Source: CAD feature listing. Evaluate the final solid. Frame: model axes, mm. A direction names the side the tool comes from. Give positions to 0.01 mm unless a question says otherwise; leave off trailing zeros. Order: outer loops, then holes, each group sorted by start corner. A loop starts at its lowest first (then second) coordinate and runs counter-clockwise, first axis right, second up.
Autodesk Inventor part; units mm, degrees
ref_plane "YZ Plane" through (0, 0, 0) normal (1, 0, 0) x (0, 1, 0)
ref_plane "XZ Plane" through (0, 0, 0) normal (0, 1, 0) x (-1, 0, 0)
ref_plane "XY Plane" through (0, 0, 0) normal (0, 0, 1) x (1, 0, 0)
sketch "Sketch1" plane through (0, 0, 0) normal (0, 0, 1) x (1, 0, 0)
  line L0 (-60.5, 11) -> (-54, 11)
  line L1 (-54, 11) -> (-54, 9)
  line L2 (-54, 9) -> (54, 9)
  line L3 (54, 9) -> (54, 11)
  line L4 (54, 11) -> (60.5, 11)
  line L5 (60.5, 11) -> (60.5, 22)
  line L6 (60.5, 22) -> (58.5, 22)
  line L7 (58.5, 22) -> (52.5, 16)
  line L8 (52.5, 16) -> (-52.5, 16)
  line L9 (-52.5, 16) -> (-58.5, 22)
  line L10 (-58.5, 22) -> (-60.5, 22)
  line L11 (-60.5, 22) -> (-60.5, 11)
  line L12 (-84.7, 0) -> (84.7, 0)
  point P0 (0, 0)
  point P1 (0, 16)
  point P2 (0, 9)
  dimension "d0" = 11
  dimension "d1" = 6.5
  dimension "d2" = 9
  dimension "d4" = 105
  dimension "d6" = 2
  dimension "d7" = 16
  dimension "d8" = 22
revolve "Revolution1" add sketch "Sketch1" angle 360 about axis through (-10, 0, 0) along (1, 0, 0)
properties part number "Riiserolle"
1) First-contact query: pin 1 Ø2 at (x, y) = (-46, 1) entering from +Z; pin 2 Ø6 at (x, z) = (40, 8) entering from -Y; pin 3 Ø17.5 at (y, z) = (5, 3.5) entering from -X; pin 4 Ø8 at (x, z) = (27.5, -10) entering from -Y. Flat tips, straight axial feed; report the tip coordinate or a pass-through.
Checks:
pin 1: stops at z = 16
pin 2: stops at y = -15.2
pin 3: stops at x = -60.5
pin 4: stops at y = -14.83
2) Section query C-C on x = 40. Output: boundary loops of the cut face in (y, z).
Checks:
outline: circle Ø32 at (0, 0); hole circle Ø18 at (0, 0)
3) Section query A-A on z = 0. Output: boundary loops of the cut face in (x, y), and give its area (3 significant figures).
Checks:
outline: (-60.5, -22) - (-58.5, -22) - (-52.5, -16) - (52.5, -16) - (58.5, -22) - (60.5, -22) - (60.5, -11) - (54, -11) - (54, -9) - (-54, -9) - (-54, -11) - (-60.5, -11) - close; (-60.5, 11) - (-54, 11) - (-54, 9) - (54, 9) - (54, 11) - (60.5, 11) - (60.5, 22) - (58.5, 22) - (52.5, 16) - (-52.5, 16) - (-58.5, 22) - (-60.5, 22) - close
area: 1,760 mm2
4) Pull-direction query (Z, two-part tool) for faces 1 (the face through (-59.514, -4.769, 21.477)), 2 (the face through (0.756, -1.172, 8.923)), 3 (the face through (60.5, 5, 10)); classes: +Z half, -Z half, draft (parallel to the pull), parting line (faces both ways), or undercut.
Checks:
face 1: parting line
face 2: undercut
face 3: draft
5) Reachability of faces 4 (the face through (57.3, -2.38, -10.74)), 5 (the face through (-60.5, 5, 10)), 6 (the face through (-57.2, -2.38, -10.74)), 7 (the face through (-52.875, 15.619, -4.919)) from +Z, -Z, +X, -X, +Y, -Y: full face, straight path, thin tool, end or side. Return the list, or none.
Checks:
face 4: +X
face 5: +Z, -Z, -X, +Y, -Y
face 6: -X
face 7: none
6) Ray query, L1, parallel to Z at x = 22, y = 0; L2, parallel to Z at x = 17, y = 3.5; L3, parallel to Y at x = 6.5, z = 7. Return the intervals inside material, ascending.
Checks:
L1: z = -16 to -9, 9 to 16
L2: z = -15.61 to -8.29, 8.29 to 15.61
L3: y = -14.39 to -5.66, 5.66 to 14.39
